```python
from build123d import *

# Parameters (mm, degrees)
F1_DEPTH = 1
F3_R     = 5


with BuildPart() as f1:
    # F0 (on Top) → F1 (new body, symmetric)
    with BuildSketch(Plane.XY):
        with BuildLine():
            Line((-4.541901, -1.5), (5.087722, -1.5))
            ThreePointArc((5.087722, -1.5), (11.75, 0), (5.087722, 1.5))
            Line((5.087722, 1.5), (-4.541901, 1.5))
            ThreePointArc((-4.541901, 1.5), (-12.25, 0), (-4.541901, -1.5))
        make_face()
        with BuildLine():
            ThreePointArc((-6.175, 0), (-8.25, -2.075), (-10.325, 0))
            Line((-10.325, 0), (-6.175, 0))
        make_face(mode=Mode.SUBTRACT)
        with BuildLine():
            ThreePointArc((9.9, 0), (8.25, -1.65), (6.6, 0))
            Line((6.6, 0), (9.9, 0))
        make_face(mode=Mode.SUBTRACT)
        with BuildLine():
            Line((-6.175, 0), (-10.325, 0))
            ThreePointArc((-10.325, 0), (-8.25, -2.075), (-6.175, 0))
        make_face()
        with BuildLine():
            Line((9.9, 0), (6.6, 0))
            ThreePointArc((6.6, 0), (8.25, -1.65), (9.9, 0))
        make_face()
    extrude(amount=F1_DEPTH, both=True)

    # F0 (on Top) → F2 (revolve, cut)
    with BuildSketch(Plane.XY):
        with BuildLine():
            Line((-6.175, 0), (-10.325, 0))
            ThreePointArc((-10.325, 0), (-8.25, -2.075), (-6.175, 0))
        make_face()
        with BuildLine():
            Line((9.9, 0), (6.6, 0))
            ThreePointArc((6.6, 0), (8.25, -1.65), (9.9, 0))
        make_face()
    revolve(axis=Axis((3.561865, 0, 0), (1, 0, 0)), mode=Mode.SUBTRACT)

    # F3
    f3_edges = [f1.edges().sort_by_distance(p)[0] for p in [
        (-4.541901, 1.5, 0),
        (5.087722, 1.5, 0),
        (-4.541901, -1.5, 0),
        (5.087722, -1.5, 0),
    ]]
    fillet(f3_edges, radius=F3_R)


solid = f1.part
```
Geometry check sheet. Reference: the model listing, model coordinates, mm. A direction names the side the tool comes from. Give positions to 0.01 mm unless a question says otherwise; leave off trailing zeros. Order: outer loops, then holes, each group sorted by start corner. A loop starts at its lowest first (then second) coordinate and runs counter-clockwise, first axis right, second up. Notation, with made-up numbers: (52.25, -33) - (91.25, -33) arc R22 ccw to (91.25, -22) - close; hole circle Ø10 at (50.5, -2). An arc over 180 degrees is marked (long way). Answer in a Markdown table with one row per item. Add a question column.
Q1. Material ranges on probe 1 along Y at (x, z) = (-7.75, -0.7); probe 2 along Z at (x, y) = (10.75, 0.25); probe 3 along Y at (x, z) = (-7.25, -0.65), recorded low to high. Write a range as from..to.
Q2. Cross-section at B-B, the plane x = -8. Enter the section's corners in (y, z).
Q3. Cross-section at D-D, the plane x = -1.5. Enter the section's corners in (y, z).
Q4. Gauge pin test, flat ends, axial feed: pin 1 (2 mm diameter, centred on x = 8, z = 1, fed in from -Y); pin 2 (1 mm diameter, centred on x = 0.5, z = 0, fed in from +Y); pin 3 (3 mm diameter, centred on x = 3.5, y = -3, fed in from -Z). Record the tip position at first contact, or that the pin passes through.
Q5. Cross-section at A-A, the plane y = 0.5. Enter the section's corners in (x, z), then the cut area to 3 significant figures.
Q6. Mould release check, pull along X, two halves, no side actions. Record for faces 1 (the flat face through (0, 0, 1)), 2 (the cylindrical face through (4.51, 1.81, 0.01)): pulls with the +X half, pulls with the -X half, needs draft (parallel to the pull), parting line crosses it, or undercut.
Q7. Tool access check on faces 3 (the cylindrical face through (11.75, -0.11, 0.01)), 4 (the flat face through (0, 1.5, 0)), 5 (the flat face through (0, -1.5, 0)). Record the directions out of +Z, -Z, +X, -X, +Y, -Y that give a thin tool (end or side, any length) a straight path to the whole face; none if there is none.
Q8. Cross-section at C-C, the plane z = 0.7. Enter the section's corners in (x, y), then the cut area to 3 significant figures.
Check values:
| question | item | result |
|---|---|---|
| 1 | probe 1 | y = -3.97..-1.89, 1.89..3.97 |
| 1 | probe 2 | z = -1..1 |
| 1 | probe 3 | y = -3.87..-1.7, 1.7..3.87 |
| 2 | outline | (-3.99, -1) - (-1.8, -1) arc R2.06 cw to (-1.8, 1) - (-3.99, 1) - close; (1.8, -1) - (3.99, -1) - (3.99, 1) - (1.8, 1) arc R2.06 cw to start |
| 3 | outline | (-1.5, -1) - (1.5, -1) - (1.5, 1) - (-1.5, 1) - close |
| 4 | pin 1 | stops at y = -3.5 |
| 4 | pin 2 | stops at y = 1.5 |
| 4 | pin 3 | stops at z = -1 |
| 5 | outline | (-12.22, -1) - (-10, -1) arc R2.01 cw to (-10, 1) - (-12.22, 1) - close; (-6.5, -1) - (7.04, -1) arc R1.57 cw to (7.04, 1) - (-6.5, 1) arc R2.01 cw to start; (9.46, -1) - (11.71, -1) - (11.71, 1) - (9.46, 1) arc R1.57 cw to start |
| 5 | area | 34.3 mm^2 |
| 6 | face 1 | needs draft |
| 6 | face 2 | undercut |
| 7 | face 3 | +Z, -Z |
| 7 | face 4 | +Z, -Z, +Y |
| 7 | face 5 | +Z, -Z, -Y |
| 8 | outline | (-5.48, -2.89) arc R5 cw to (-2.03, -1.5) - (2.77, -1.5) arc R5 cw to (5.99, -2.68) arc R3.5 ccw (long way) to (5.99, 2.68) arc R5 cw to (2.77, 1.5) - (-2.03, 1.5) arc R5 cw to (-5.48, 2.89) arc R4 ccw (long way) to start; hole circle Ø3.91 at (-8.25, 0); hole circle Ø2.99 at (8.25, 0) |
| 8 | area | 100 mm^2 |
